```python
from build123d import *

# Parameters (mm, degrees)
SKETCH1_R           = 13.49375
SKETCH1_R_2         = 12.7
BOSS_EXTRUDE1_DEPTH = 50.8
CUT_EXTRUDE1_DEPTH  = 55.266035217


with BuildPart() as part:
    # Sketch1 → Boss-Extrude1 (new body)
    with BuildSketch(Plane.XY):
        Circle(SKETCH1_R)
        Circle(SKETCH1_R_2, mode=Mode.SUBTRACT)
    extrude(amount=BOSS_EXTRUDE1_DEPTH)

    # Sketch2 → Cut-Extrude1 (cut, through all)
    with BuildSketch(Plane.XY.offset(50.8)):
        with BuildLine():
            Line((0, 0), (0, 13.49375))
            ThreePointArc((0, 13.49375), (0.588589108, 13.48090694), (1.176057804, 13.442402207))
            Line((1.176057804, 13.442402207), (0, 0))
        make_face()
    extrude(amount=-CUT_EXTRUDE1_DEPTH, mode=Mode.SUBTRACT)


solid = part.part
```
Work out the finished part from the listing and answer in its coordinate system (mm). Round coordinates to 2 decimals unless told otherwise and drop trailing zeros. Order: outer loops, then holes, each group sorted by start corner. A loop starts at its lowest first (then second) coordinate and runs counter-clockwise, first axis right, second up.
Q1. Find the intervals of material crossed by line 1 along X through (y, z) = (0, 25.5); line 2 along Y through (x, z) = (-9.5, 37); line 3 along X through (y, z) = (-6.5, 43), in increasing order.
Solution:
line 1: x = -13.49 to -12.7, 12.7 to 13.49
line 2: y = -9.58 to -8.43, 8.43 to 9.58
line 3: x = -11.83 to -10.91, 10.91 to 11.83
Q2. A cutting plane is placed at B-B, the plane y = -3.75. Determine the outline of the cut face in (x, z), then the cut area to 3 significant figures.
Solution:
outline: (-12.96, 0) - (-12.13, 0) - (-12.13, 50.8) - (-12.96, 50.8) - close; (12.13, 0) - (12.96, 0) - (12.96, 50.8) - (12.13, 50.8) - close
area: 84.2 mm2
Q3. A cutting plane is placed at C-C, the plane z = 3.5. Determine the outline of the cut face in (x, y), then the cut area to 3 significant figures.
Solution:
outline: (0, 12.7) - (0, 13.49) arc R13.49 ccw (long way) to (1.18, 13.44) - (1.11, 12.65) arc R12.7 cw (long way) to start
area: 64.4 mm2
Q4. Given pin 1 Ø10 at (x, z) = (6.5, 24.5) entering from +Y; pin 2 Ø2 at (y, z) = (-8, 35.5) entering from +X; pin 3 Ø6 at (y, z) = (-11, 39.5) entering from -X, each flat-ended and moving along its own axis, determine where each tip first touches the part or whether it passes through.
Solution:
pin 1: stops at y = 13.41
pin 2: stops at x = 11.54
pin 3: stops at x = -10.87
Q5. A cutting plane is placed at A-A, the plane x = 5.5. Determine the outline of the cut face in (y, z).
Solution:
outline: (-12.32, 0) - (-11.45, 0) - (-11.45, 50.8) - (-12.32, 50.8) - close; (11.45, 0) - (12.32, 0) - (12.32, 50.8) - (11.45, 50.8) - close
